```python
from build123d import *

# Parameters (mm, degrees)
SKETCH1_R           = 2.395
BOSS_EXTRUDE1_DEPTH = 3
SKETCH2_R           = 2.365
BOSS_EXTRUDE2_DEPTH = 3


with BuildPart() as part:
    # Sketch1 → Boss-Extrude1 (new body)
    with BuildSketch(Plane.XY):
        with BuildLine():
            Line((0, 3), (20, 3))
            ThreePointArc((20, 3), (23, 0), (20, -3))
            Line((20, -3), (0, -3))
            ThreePointArc((0, -3), (-3, 0), (0, 3))
        make_face()
        Circle(SKETCH1_R, mode=Mode.SUBTRACT)
        with Locations((20, 0)):
            Circle(SKETCH1_R, mode=Mode.SUBTRACT)
    extrude(amount=BOSS_EXTRUDE1_DEPTH)

    # Sketch2 → Boss-Extrude2 (add)
    with BuildSketch(Plane.XY.offset(3)):
        with BuildLine():
            Line((0.05, 3.75), (19.95, 3.75))
            ThreePointArc((19.95, 3.75), (23.7, 0), (19.95, -3.75))
            Line((19.95, -3.75), (0.05, -3.75))
            ThreePointArc((0.05, -3.75), (-3.7, 0), (0.05, 3.75))
        make_face()
        Circle(SKETCH2_R, mode=Mode.SUBTRACT)
        with Locations((20, 0)):
            Circle(SKETCH2_R, mode=Mode.SUBTRACT)
    extrude(amount=-BOSS_EXTRUDE2_DEPTH)


solid = part.part
```
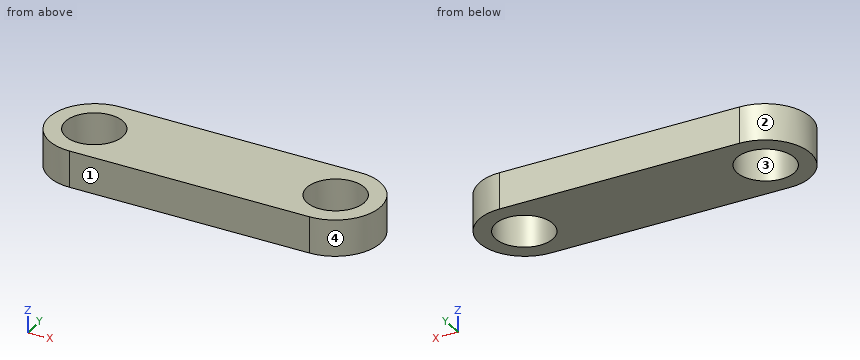
For this review, take the finished solid that the model builds, in its own axes (mm). Face numbers are marked on the shaded views. Coordinates: 2 decimals unless noted, no trailing zeros. Loops run counter-clockwise (first coordinate to the right, second up) from the corner with the lowest first, then second, coordinate; pieces in that order, holes last. Notation, with made-up numbers: (73, 79.5) -> (78, 79.5) arc R18 cw to (78, 111.5) -> close; hole circle Ø4 at (61, 63.5). An arc over 180 degrees is marked (long way). Return JSON: item names as keys, results as strings. Group by question number.
(1) Consider section D-D, the plane y = -3. Give the boundary of the cut face in (x, z).
(2) Mouldability with a two-part tool opening along X and no side actions: class the marked faces 1, 2, 3 and 4 as pulls with the +X half, pulls with the -X half, needs draft (parallel to the pull), parting line crosses it, or undercut.
(3) To check wall thickness, follow L1, parallel to X at y = 1.5, z = 0.7; L2, parallel to Y at x = 0, z = 2.3 (3 decimals); L3, parallel to X at y = -1.75, z = 0.8. State the ranges of each line that lie inside material, in increasing order.
(4) Consider section A-A, the plane y = 0. Give the boundary of the cut face in (x, z) (3 decimals), plus the area to 3 significant figures.
(5) Consider section C-C, the plane x = 21. Give the boundary of the cut face in (y, z), plus the area to 3 significant figures.
(6) Consider section B-B, the plane z = 0.9. Give the boundary of the cut face in (x, y) (3 decimals).
Results below:
{
 "1": {"outline": "(-2.2, 0) -> (22.2, 0) -> (22.2, 3) -> (-2.2, 3) -> close"},
 "2": {"face 1": "needs draft", "face 2": "pulls with the -X half", "face 3": "undercut", "face 4": "pulls with the +X half"},
 "3": {"L1": "x = -3.39 to -1.83, 1.83 to 18.17, 21.83 to 23.39", "L2": "y = -3.75 to -2.365, 2.365 to 3.75", "L3": "x = -3.27 to -1.59, 1.59 to 18.41, 21.59 to 23.27"},
 "4": {"outline": "(-3.7, 0) -> (-2.365, 0) -> (-2.365, 3) -> (-3.7, 3) -> close; (2.365, 0) -> (17.635, 0) -> (17.635, 3) -> (2.365, 3) -> close; (22.365, 0) -> (23.7, 0) -> (23.7, 3) -> (22.365, 3) -> close", "area": "53.8 mm2"},
 "5": {"outline": "(-3.6, 0) -> (-2.14, 0) -> (-2.14, 3) -> (-3.6, 3) -> close; (2.14, 0) -> (3.6, 0) -> (3.6, 3) -> (2.14, 3) -> close", "area": "8.74 mm2"},
 "6": {"outline": "(0.05, -3.75) -> (19.95, -3.75) arc R3.75 ccw to (19.95, 3.75) -> (0.05, 3.75) arc R3.75 ccw to start; hole circle Ø4.73 at (0, 0); hole circle Ø4.73 at (20, 0)"}
}
